from build123d import *

# Parameters (mm, degrees)
ESQUISSE1_R             = 12.8
ESQUISSE1_R_2           = 2
ESQUISSE1_R_3           = 1.55
BOSS_EXTRU_1_DEPTH      = 1.6
ESQUISSE2_R             = 0.5
ENL_V_MAT_EXTRU_1_DEPTH = 19.172506707
ENL_V_MAT_EXTRU_2_DEPTH = 0.4


with BuildPart() as part:
    # Esquisse1 → Boss.-Extru.1 (new body)
    with BuildSketch(Plane.XY):
        Circle(ESQUISSE1_R)
        Circle(ESQUISSE1_R_2, mode=Mode.SUBTRACT)
        with Locations((-11, 0)):
            Circle(ESQUISSE1_R_3, mode=Mode.SUBTRACT)
        with Locations((11, 0)):
            Circle(ESQUISSE1_R_3, mode=Mode.SUBTRACT)
    extrude(amount=BOSS_EXTRU_1_DEPTH)

    # Esquisse2 → Enlèv. mat.-Extru.1 (cut, through all)
    with BuildSketch(Plane.XY.offset(1.6)):
        with Locations((5, -7.765166341)):
            Circle(ESQUISSE2_R)
        with Locations((-5, -7.765166341)):
            Circle(ESQUISSE2_R)
        with Locations((0, 7.998956295)):
            Circle(ESQUISSE2_R)
        with Locations((5, 7.998956295)):
            Circle(ESQUISSE2_R)
        with Locations((-5, 7.998956295)):
            Circle(ESQUISSE2_R)
    extrude(amount=-ENL_V_MAT_EXTRU_1_DEPTH, mode=Mode.SUBTRACT)

    # Esquisse4 → Enlèv. mat.-Extru.2 (cut)
    with BuildSketch(Plane.XY.offset(1.6)):
        with BuildLine():
            Line((2.849870715, 13.22379947), (4.768486358, 12.659074744))
            Line((4.768486358, 12.659074744), (3.524647017, 8.433211229))
            ThreePointArc((3.524647017, 8.433211229), (3.562251348, 7.452950263), (4.184819655, 6.694837904))
            ThreePointArc((4.184819655, 6.694837904), (6.905555582, 3.827123228), (7.895161183, 0))
            ThreePointArc((7.895161183, 0), (8.427320022, -1.738200739), (9.8413761, -2.88055806))
            Line((9.8413761, -2.88055806), (13.173167165, -4.220677813))
            Line((13.173167165, -4.220677813), (12.426832835, -6.076206058))
            Line((12.426832835, -6.076206058), (9.09504177, -4.736086305))
            ThreePointArc((9.09504177, -4.736086305), (6.770113236, -2.857872865), (5.895161183, 0))
            ThreePointArc((5.895161183, 0), (5.156242193, 2.857637453), (3.124722322, 4.998903458))
            ThreePointArc((3.124722322, 4.998903458), (1.692538076, 6.742899364), (1.606031374, 8.997935955))
            Line((1.606031374, 8.997935955), (2.849870715, 13.22379947))
        make_face()
        Polygon((-3.439832578, 13.22379947), (-1.439832578, 13.22379947), (-1.439832578, 5.505940762), (1, 0.219636844), (1, -13.772678102), (-1, -13.772678102), (-1, -0.219636844), (-3.439832578, 5.066667074), align=None)
    extrude(amount=-ENL_V_MAT_EXTRU_2_DEPTH, mode=Mode.SUBTRACT)


solid = part.part
Can you work these out from the model? Positions are in its coordinate system, mm. A direction names the side the tool comes from. Give positions to 0.01 mm unless a question says otherwise; leave off trailing zeros. Order: outer loops, then holes, each group sorted by start corner. A loop starts at its lowest first (then second) coordinate and runs counter-clockwise, first axis right, second up. Notation, with made-up numbers: M 20.25,44.25 L 41.25,44.25 A31 cw 41.25,76.25 Z; hole C 61.5,29 d10. An arc over 180 degrees is marked long. One line per question, with ' | ' between items.
Item 1: Please list where these lines run through material, in increasing order: L1, parallel to Y at x = 0, z = 0.6; L2, parallel to X at y = 1, z = 0.85; L3, parallel to Y at x = -5, z = 1.
Answer block:
L1: y = -12.8 to -2, 2 to 7.5, 8.5 to 12.8 | L2: x = -12.76 to -12.18, -9.82 to -1.73, 1.73 to 9.82, 12.18 to 12.76 | L3: y = -11.78 to -8.27, -7.27 to 7.5, 8.5 to 11.78
Item 2: I'm going to push a flat-ended pin straight in: pin 1 Ø2.5 at (x, y) = (-11, 0) entering from +Z. Where does the tip first touch, or does it pass through?
Answer block:
pin 1: passes through
Item 3: We'd pull the mould along X, two halves only. Please class faces 1 (the face through (8.4, -1.7, 1.4)), 2 (the face through (-7, 0, 1.6)), 3 (the face through (-10.158, -7.789, 0.789)): released by +X, released by -X, zero draft, split by the parting line, or undercut.
Answer block:
face 1: undercut | face 2: zero draft | face 3: split by the parting line
Item 4: Suppose I cut it at A-A, the plane x = 5. Write out the boundary of the cut face in (y, z).
Answer block:
outline: M -11.78,0 L -8.27,0 L -8.27,1.6 L -11.78,1.6 Z; M -7.27,0 L 7.5,0 L 7.5,1.6 L 6.11,1.6 L 6.11,1.2 L 3.12,1.2 L 3.12,1.6 L -7.27,1.6 Z; M 8.5,0 L 11.78,0 L 11.78,1.6 L 8.5,1.6 Z
Item 5: Suppose I cut it at D-D, the plane y = 4.5. Write out the boundary of the cut face in (x, z).
Answer block:
outline: M -11.98,0 L 11.98,0 L 11.98,1.6 L 6.49,1.6 L 6.49,1.2 L 3.81,1.2 L 3.81,1.6 L -0.98,1.6 L -0.98,1.2 L -3.18,1.2 L -3.18,1.6 L -11.98,1.6 Z
Item 6: Suppose I cut it at B-B, the plane x = -11. Write out the boundary of the cut face in (y, z).
Answer block:
outline: M -6.55,0 L -1.55,0 L -1.55,1.6 L -6.55,1.6 Z; M 1.55,0 L 6.55,0 L 6.55,1.6 L 1.55,1.6 Z
Item 7: Suppose I cut it at C-C, the plane z = 0.95. Give the number of separate pieces and of enclosed holes in the cut face, then the cut area to 3 significant figures.
Answer block:
separate pieces: 1 | enclosed holes: 8 | area: 483 mm2
Item 8: For faces 4 (the face through (0, -7, 1.2)), 5 (the face through (-0.64, 3.77, 1.4)), 6 (the face through (10.3, -5.22, 1.4)), which set-ups out of +Z, -Z, +X, -X, +Y, -Y let a thin tool reach every point of the face, with its end or its side?
Answer block:
face 4: +Z, -Y | face 5: +Z | face 6: +Z, +X
